```python
from build123d import *

# Parameters (mm, degrees)
SKETCH_1_W          = 70
SKETCH_1_H          = 20
EXTRUDE_1_DEPTH     = 5
SKETCH_2_R          = 1.9
CUT_EXTRUDE_1_DEPTH = 5
SKETCH_3_W          = 25
SKETCH_3_H          = 10
EXTRUDE_2_DEPTH     = 10
SKETCH_4_W          = 15
SKETCH_4_H          = 10
CUT_EXTRUDE_2_DEPTH = 10
SKETCH_5_R          = 1.9
CUT_EXTRUDE_3_DEPTH = 56.509008278


with BuildPart() as part:
    # ｽｹｯﾁ1 → ﾎﾞｽ - 押し出し1 (new body)
    with BuildSketch(Plane.XY):
        Rectangle(SKETCH_1_W, SKETCH_1_H)
    extrude(amount=EXTRUDE_1_DEPTH)

    # ｽｹｯﾁ2 → ｶｯﾄ - 押し出し1 (cut)
    with BuildSketch(Plane.XY.offset(5)):
        with Locations((-30, 5)):
            Circle(SKETCH_2_R)
        with Locations((-30, -5)):
            Circle(SKETCH_2_R)
        with Locations((30, 5)):
            Circle(SKETCH_2_R)
        with Locations((30, -5)):
            Circle(SKETCH_2_R)
    extrude(amount=-CUT_EXTRUDE_1_DEPTH, mode=Mode.SUBTRACT)

    # ｽｹｯﾁ3 → ﾎﾞｽ - 押し出し2 (add)
    with BuildSketch(Plane.XY.offset(5)):
        with Locations((-5, 0)):
            Rectangle(SKETCH_3_W, SKETCH_3_H)
    extrude(amount=EXTRUDE_2_DEPTH)

    # ｽｹｯﾁ4 → ｶｯﾄ - 押し出し2 (cut)
    with BuildSketch(Plane.XY.offset(15)):
        with Locations((-5, 0)):
            Rectangle(SKETCH_4_W, SKETCH_4_H)
    extrude(amount=-CUT_EXTRUDE_2_DEPTH, mode=Mode.SUBTRACT)

    # ｽｹｯﾁ5 → ｶｯﾄ - 押し出し3 (cut, through all)
    with BuildSketch(Plane.ZY.offset(17.5)):
        with Locations((10, 0)):
            Circle(SKETCH_5_R)
    extrude(amount=-CUT_EXTRUDE_3_DEPTH, mode=Mode.SUBTRACT)


solid = part.part
```
For this review, take the finished solid that the model builds, in its own axes (mm). A direction names the side the tool comes from. Give positions to 0.01 mm unless a question says otherwise; leave off trailing zeros. Write each loop counter-clockwise with the first axis right and the second up, starting at its lowest first coordinate (ties: lowest second). Pieces come first, ordered by that corner, then holes.
Item 1: Wall thickness on probe 1 along Y at (x, z) = (-30, 3.85); probe 2 along X at (y, z) = (3.25, 9.25); probe 3 along Y at (x, z) = (6, 10): over which ranges is each line inside the solid? List them lowest first.
Item 2: Take a section at D-D (x = -14.5). Give the boundary of the cut face in (y, z), and give its area (3 significant figures).
Item 3: Insertion check: P1, Ø5.5, axis at x = 6, z = 9, coming from the +Y side; P2, Ø4, axis at x = 20.5, y = 6, coming from the -Z side; P3, Ø3, axis at x = -30, y = 5, coming from the -Z side; P4, Ø5.5, axis at x = -15.5, z = 12, coming from the -Y side. Each pin has a flat end and moves straight along its axis. Give the tip position at first contact, or say it passes through.
Item 4: The part is to be moulded in two halves that separate along Z. For faces 6 (the face through (4.965, -0.728, 11.755)), 7 (the face through (0, -10, 2)), 8 (the face through (0, 0, 0)), 9 (the face through (-15.035, -0.728, 11.755)), say which applies: +Z half, -Z half, draft (parallel to the pull), parting line (faces both ways), or undercut.
Item 5: Take a section at B-B (x = -30). Give the boundary of the cut face in (y, z).
Item 6: Take a section at C-C (z = 1). Give the boundary of the cut face in (x, y), and give its area (3 significant figures).
Item 7: Take a section at A-A (z = 10). Give the boundary of the cut face in (x, y), and give its area (3 significant figures).
Item 8: Machinability: for faces 1 (the face through (5, -5, 10)), 2 (the face through (7.5, -0.1, 12.2)), 3 (the face through (-17.5, -0.1, 12.2)), 4 (the face through (-12.5, -0.1, 7.8)), 5 (the face through (-15, 5, 10)), which of the approach directions +Z, -Z, +X, -X, +Y, -Y give a long, thin tool a straight path to every point of the face, cutting with its end or side? Answer none if there is none.
Established:
1. probe 1: y = -10 to -6.9, -3.1 to 3.1, 6.9 to 10
1. probe 2: x = -17.5 to -12.5, 2.5 to 7.5
1. probe 3: y = -5 to -1.9, 1.9 to 5
2. outline: (-10, 0) - (10, 0) - (10, 5) - (5, 5) - (5, 15) - (-5, 15) - (-5, 5) - (-10, 5) - close; hole circle Ø3.8 at (0, 10)
2. area: 189 mm2
3. P1: stops at y = 5
3. P2: stops at z = 0
3. P3: passes through
3. P4: stops at y = -5
4. face 6: undercut
4. face 7: draft
4. face 8: -Z half
4. face 9: undercut
5. outline: (-10, 0) - (-6.9, 0) - (-6.9, 5) - (-10, 5) - close; (-3.1, 0) - (3.1, 0) - (3.1, 5) - (-3.1, 5) - close; (6.9, 0) - (10, 0) - (10, 5) - (6.9, 5) - close
6. outline: (-35, -10) - (35, -10) - (35, 10) - (-35, 10) - close; hole circle Ø3.8 at (-30, -5); hole circle Ø3.8 at (-30, 5); hole circle Ø3.8 at (30, -5); hole circle Ø3.8 at (30, 5)
6. area: 1,350 mm2
7. outline: (-17.5, -5) - (-12.5, -5) - (-12.5, -1.9) - (-17.5, -1.9) - close; (-17.5, 1.9) - (-12.5, 1.9) - (-12.5, 5) - (-17.5, 5) - close; (2.5, -5) - (7.5, -5) - (7.5, -1.9) - (2.5, -1.9) - close; (2.5, 1.9) - (7.5, 1.9) - (7.5, 5) - (2.5, 5) - close
7. area: 62.0 mm2
8. face 1: +Z, +X, -X, -Y
8. face 2: +Z, +X, +Y, -Y
8. face 3: +Z, -X, +Y, -Y
8. face 4: +Z, +Y, -Y
8. face 5: +Z, +X, -X, +Y
